Could you check a few things on this model? Use its own coordinates, in mm. A direction names the side the tool comes from. Round coordinates to 2 decimals unless told otherwise and drop trailing zeros. Order: outer loops, then holes, each group sorted by start corner. A loop starts at its lowest first (then second) coordinate and runs counter-clockwise, first axis right, second up.
Autodesk Inventor part; units mm, degrees
ref_plane "YZ Plane" through (0, 0, 0) normal (1, 0, 0) x (0, 1, 0)
ref_plane "XZ Plane" through (0, 0, 0) normal (0, 1, 0) x (-1, 0, 0)
ref_plane "XY Plane" through (0, 0, 0) normal (0, 0, 1) x (1, 0, 0)
sketch "スケッチ1" plane through (0, 0, 0) normal (0, 0, 1) x (1, 0, 0)
  line L0 (0, 0) -> (20, 0)
  line L1 (20, 0) -> (20, 158)
  line L2 (20, 158) -> (0, 158)
  line L3 (0, 158) -> (0, 0)
  dimension "d0" = 158
  dimension "d1" = 20
extrude "押し出し1" add sketch "スケッチ1" along normal blind 3
sketch "スケッチ2" plane through (0, 0, 3) normal (0, 0, 1) x (1, 0, 0)
  line L0 (0, 0) -> (20, 0)
  line L1 (20, 0) -> (20, 158)
  point P0 (10, 138)
  point P1 (10, 20)
  dimension "d4" = 20
  dimension "d5" = 118
  dimension "d6" = 10
  dimension "d7" = 10
hole "穴1" at (10, 138, 3) at (10, 20, 3) direction (0, 0, -1) diameter 3.2 depth 8
sketch "スケッチ3" plane through (0, 0, 3) normal (0, 0, 1) x (1, 0, 0)
  circle A0 centre (10, 20) radius 1.6
  circle A1 centre (10, 138) radius 1.6
  line L0 (20, 0) -> (20, 158)
  line L1 (20, 158) -> (0, 158)
  line L2 (0, 158) -> (0, 0)
  line L3 (0, 0) -> (20, 0)
  circle A2 centre (10, 138) radius 3
  circle A3 centre (10, 20) radius 3
  dimension "d15" = 6
  dimension "d16" = 6
extrude "押し出し2" cut sketch "スケッチ3" against normal blind 2 contours A1 | A2 | A3
fillet "フィレット1" radius 5 4 edges at (0, 158, 1.5) (20, 158, 1.5) (0, 0, 1.5) (20, 0, 1.5)
equation "\"d16\" = d15"
properties part number "BP_BOX-Bar"
Q1. We'd pull the mould along X, two halves only. Please class faces 3 (the flat face through (20, 78, 1)), 4 (the flat face through (10, 80, 3)), 5 (the flat face through (11.3, 18.7, 1)): released by +X, released by -X, zero draft, split by the parting line, or undercut.
Q2. For P1, Ø5, axis at x = 10, y = 138, coming from the +Z side, with a flat end and sliding along its axis, tell me the tip position at first contact or that it passes through.
Q3. Imagine slicing it at B-B, the plane x = 10. Please give me the cut outline in (y, z).
Q4. I need wall thicknesses on L1, parallel to Y at x = 10, z = 0.4; L2, parallel to Y at x = 10, z = 2.05; L3, parallel to X at y = 138, z = 0.85. Which ranges of each line are inside material? Lowest first, please.
Q5. Imagine slicing it at C-C, the plane y = 138. Please give me the cut outline in (x, z), then the cut area to 3 significant figures.
Q6. Imagine slicing it at A-A, the plane z = 1.9. Please give me the cut outline in (x, y).
Q7. For faces 1 (the flat face through (10, 0, 1)), 2 (the flat face through (11.3, 136.7, 1)), which set-ups out of +Z, -Z, +X, -X, +Y, -Y let a thin tool reach every point of the face, with its end or its side?
Filled in:
1. face 3: released by +X
1. face 4: zero draft
1. face 5: undercut
2. P1: stops at z = 1
3. outline: (0, 0) - (18.4, 0) - (18.4, 1) - (17, 1) - (17, 3) - (0, 3) - close; (21.6, 0) - (136.4, 0) - (136.4, 1) - (135, 1) - (135, 3) - (23, 3) - (23, 1) - (21.6, 1) - close; (139.6, 0) - (158, 0) - (158, 3) - (141, 3) - (141, 1) - (139.6, 1) - close
4. L1: y = 0 to 18.4, 21.6 to 136.4, 139.6 to 158
4. L2: y = 0 to 17, 23 to 135, 141 to 158
4. L3: x = 0 to 8.4, 11.6 to 20
5. outline: (0, 0) - (8.4, 0) - (8.4, 1) - (7, 1) - (7, 3) - (0, 3) - close; (11.6, 0) - (20, 0) - (20, 3) - (13, 3) - (13, 1) - (11.6, 1) - close
5. area: 44.8 mm2
6. outline: (0, 5) arc R5 ccw to (5, 0) - (15, 0) arc R5 ccw to (20, 5) - (20, 153) arc R5 ccw to (15, 158) - (5, 158) arc R5 ccw to (0, 153) - close; hole circle Ø6 at (10, 20); hole circle Ø6 at (10, 138)
7. face 1: +Z, -Z, +X, -X, -Y
7. face 2: +Z
